Part model, mm, in its own coordinate system. Face numbers are marked on the shaded views. A direction names the side the tool comes from. Round coordinates to 2 decimals unless told otherwise and drop trailing zeros. Write each loop counter-clockwise with the first axis right and the second up, starting at its lowest first coordinate (ties: lowest second). Pieces come first, ordered by that corner, then holes.
1) Saw through at B-B on z = 0. Write the cut outline in (x, y).
2) Flat gauge pins, fed straight in: pin 1 (1.2 mm diameter, centred on x = 0, y = 0.5, fed in from +Z); pin 2 (1.5 mm diameter, centred on x = 3, z = 6, fed in from +Y); pin 3 (3 mm diameter, centred on y = -2, z = -5.5, fed in from +X). Where does each tip first touch, or does it go through?
3) Pull direction X, two halves, no side cores. Call the marked faces 3, 4, 5 and 6: +X half, -X half, draft (parallel to the pull), parting line (faces both ways), or undercut.
4) Which spindle directions (+Z, -Z, +X, -X, +Y, -Y) get a long thin tool onto all of the face, cutting with end or side? Do the marked faces 1 and 2. Say none if no direction does.
5) Saw through at A-A on y = 0. Write the cut outline in (x, z).
6) Drill centre lines: L1, parallel to Z at x = 0.25, y = 1.25; L2, parallel to Z at x = 0.75, y = -2.75; L3, parallel to Y at x = 0, z = 1.5. Where is each one in solid material? Low to high.
```python
from build123d import *

# Parameters (mm, degrees)
CUT_EXTRUDE1_START = 7.96925
CUT_EXTRUDE1_DEPTH = 2.413


with BuildPart() as part:
    # Sketch2 → Revolve1 (revolve)
    with BuildSketch(Plane(origin=(0, 0, 0), x_dir=(0, 0, -1), z_dir=(1, 0, 0)), mode=Mode.PRIVATE) as revolve1_sk:
        with BuildLine():
            Line((7.96925, 0), (7.96925, 2.2145625))
            Line((7.96925, 2.2145625), (7.7708125, 2.413))
            Line((7.7708125, 2.413), (-3.14325, 2.413))
            Line((-3.14325, 2.413), (-3.14325, 3.72745))
            ThreePointArc((-3.14325, 3.72745), (-3.213925134, 3.898074866), (-3.38455, 3.96875))
            Line((-3.38455, 3.96875), (-7.72795, 3.96875))
            ThreePointArc((-7.72795, 3.96875), (-7.898574866, 3.898074866), (-7.96925, 3.72745))
            Line((-7.96925, 3.72745), (-7.96925, 0))
            Line((-7.96925, 0), (7.96925, 0))
        make_face()
    revolve(revolve1_sk.sketch.rotate(Axis((0, 0, -7.96925), (0, 0, 1)), 90), axis=Axis((0, 0, -7.96925), (0, 0, 1)))

    # Sketch3 → Cut-Extrude1 (cut)
    with BuildSketch(Plane.XY.offset(CUT_EXTRUDE1_START)):
        Polygon((-1.984375, 1.14567944), (-1.984375, -1.14567944), (0, -2.291358881), (1.984375, -1.14567944), (1.984375, 1.14567944), (0, 2.291358881), align=None)
    extrude(amount=-CUT_EXTRUDE1_DEPTH, mode=Mode.SUBTRACT)

    # Cut-Extrude2 cone 1 section (through the dimple's axis) → Cut-Extrude2 (revolve, cut)
    with BuildSketch(Plane(origin=(0, 0, 7.96925), x_dir=(0, -1, 0), z_dir=(1, 0, 0))):
        Polygon((0, 0), (2.530707401, 0), (0, 1.461104599), align=None)
    revolve(axis=Axis((0, 0, 7.96925), (0, 0, -1)), mode=Mode.SUBTRACT)


solid = part.part
```
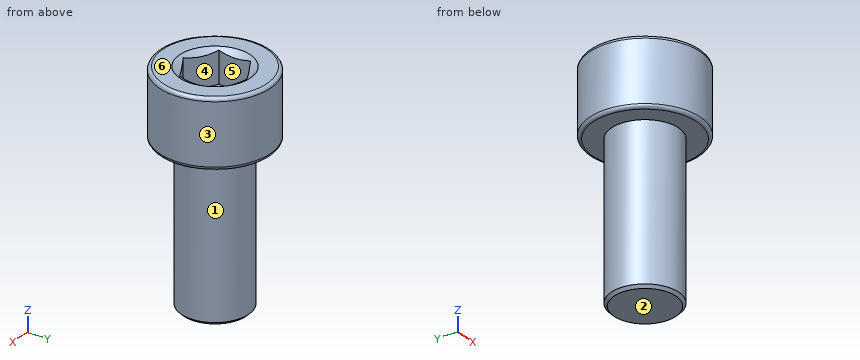
Completed:
1. outline: circle Ø4.83 at (0, 0)
2. pin 1: stops at z = 5.56
2. pin 2: stops at y = 3.27
2. pin 3: stops at x = 2.36
3. face 3: parting line
3. face 4: undercut
3. face 5: undercut
3. face 6: draft
4. face 1: -Z
4. face 2: -Z, +X, -X, +Y, -Y
5. outline: (-3.97, 3.38) arc R0.24 ccw to (-3.73, 3.14) - (-2.41, 3.14) - (-2.41, -7.77) - (-2.21, -7.97) - (2.21, -7.97) - (2.41, -7.77) - (2.41, 3.14) - (3.73, 3.14) arc R0.24 ccw to (3.97, 3.38) - (3.97, 7.73) arc R0.24 ccw to (3.73, 7.97) - (2.53, 7.97) - (1.98, 7.65) - (1.98, 5.56) - (-1.98, 5.56) - (-1.98, 7.65) - (-2.53, 7.97) - (-3.73, 7.97) arc R0.24 ccw to (-3.97, 7.73) - close
6. L1: z = -7.97 to 5.56
6. L2: z = 3.14 to 7.97
6. L3: y = -2.41 to 2.41
